For this review, take the finished solid that the model builds, in its own axes (mm). Round coordinates to 2 decimals unless told otherwise and drop trailing zeros. Order: outer loops, then holes, each group sorted by start corner. A loop starts at its lowest first (then second) coordinate and runs counter-clockwise, first axis right, second up. Notation, with made-up numbers: (-5, 77) -> (22, 77) arc R10 cw to (22, 87) -> close; hole circle Ø10 at (-18.75, -24). An arc over 180 degrees is marked (long way). Use a Markdown table: item, result. Add a question column.
1) Consider section B-B (y = 1.85). State the section outline as (x, z) points, plus the area to 3 significant figures.
2) Consider section A-A (z = 0.75). State the section outline as (x, y) points.
3) Draft analysis for pull direction Z (two halves, no side actions). For faces 1 (the face through (-18, 1, -4)), 2 (the face through (-6.5, 1.48, -0.07)), 3 (the face through (-18, 1, 4)), 4 (the face through (-26.5, 1.48, -0.07)), state which applies: pulls with the +Z half, pulls with the -Z half, needs draft (parallel to the pull), parting line crosses it, or undercut.
4) Wall thickness on line 1 along Z through (x, y) = (-28, 2.35); line 2 along X through (y, z) = (1.5, 0.75); line 3 along X through (y, z) = (0.35, -0.25): over which ranges is each line inside the solid? List them lowest first. Write a range as [from, to].
5) Consider section C-C (x = -28.5). State the section outline as (y, z) points.
6) Consider section D-D (z = -1). State the section outline as (x, y) points.
7) Clearance check with a flat-ended pin moving along its axis: P1, Ø3.5, axis at x = -28, z = 0, coming from the -Y side. State where the tip first meets the part, or that it passes through.
Autodesk Inventor part; units mm, degrees
ref_plane "YZ Plane" through (0, 0, 0) normal (1, 0, 0) x (0, 1, 0)
ref_plane "XZ Plane" through (0, 0, 0) normal (0, 1, 0) x (-1, 0, 0)
ref_plane "XY Plane" through (0, 0, 0) normal (0, 0, 1) x (1, 0, 0)
sketch "Sketch1" plane through (0, 0, 0) normal (0, 1, 0) x (-1, 0, 0)
  circle A0 centre (28, 0) radius 1.5
  circle A1 centre (8, 0) radius 1.5
  arc A2 (28, -4) -> (28, 4) centre (28, 0) ccw
  arc A3 (8, 4) -> (8, -4) centre (8, 0) ccw
  line L0 (28, 4) -> (8, 4)
  line L1 (8, -4) -> (28, -4)
  point P0 (0, 0)
  dimension "d0" = 3
  dimension "d1" = 4
  dimension "d2" = 4
  dimension "d5" = 20
extrude "Extrusion1" add sketch "Sketch1" along normal blind 3
properties part number "Light gate compression plate" material "Polycarbonate, Smoke"
Results list:
| question | item | result |
|---|---|---|
| 1 | outline | (-28, -4) -> (-8, -4) arc R4 ccw to (-8, 4) -> (-28, 4) arc R4 ccw to start; hole circle Ø3 at (-28, 0); hole circle Ø3 at (-8, 0) |
| 1 | area | 196 mm2 |
| 2 | outline | (-31.93, 0) -> (-29.3, 0) -> (-29.3, 3) -> (-31.93, 3) -> close; (-26.7, 0) -> (-9.3, 0) -> (-9.3, 3) -> (-26.7, 3) -> close; (-6.7, 0) -> (-4.07, 0) -> (-4.07, 3) -> (-6.7, 3) -> close |
| 3 | face 1 | pulls with the -Z half |
| 3 | face 2 | undercut |
| 3 | face 3 | pulls with the +Z half |
| 3 | face 4 | undercut |
| 4 | line 1 | [-4, -1.5], [1.5, 4] |
| 4 | line 2 | [-31.93, -29.3], [-26.7, -9.3], [-6.7, -4.07] |
| 4 | line 3 | [-31.99, -29.48], [-26.52, -9.48], [-6.52, -4.01] |
| 5 | outline | (0, -3.97) -> (3, -3.97) -> (3, -1.41) -> (0, -1.41) -> close; (0, 1.41) -> (3, 1.41) -> (3, 3.97) -> (0, 3.97) -> close |
| 6 | outline | (-31.87, 0) -> (-29.12, 0) -> (-29.12, 3) -> (-31.87, 3) -> close; (-26.88, 0) -> (-9.12, 0) -> (-9.12, 3) -> (-26.88, 3) -> close; (-6.88, 0) -> (-4.13, 0) -> (-4.13, 3) -> (-6.88, 3) -> close |
| 7 | P1 | y = 0 |
